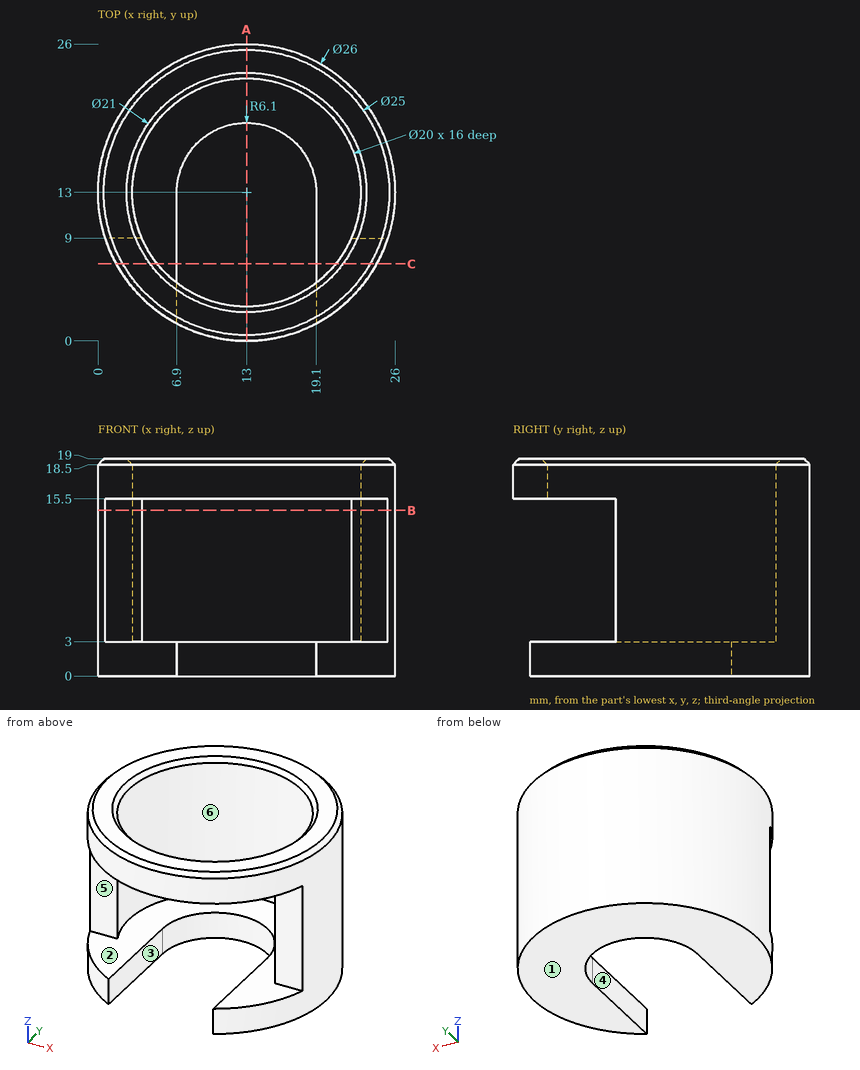
Geometry check sheet. Reference: drawing and pictorial views, mm from the part's lowest x, y, z. A direction names the side the tool comes from. Coordinates: 2 decimals unless noted, no trailing zeros. Order: outer loops, then holes, each group sorted by start corner. A loop starts at its lowest first (then second) coordinate and runs counter-clockwise, first axis right, second up. Notation, with made-up numbers: (69, 37.5) -> (127, 37.5) arc R24 ccw to (127, 54.5) -> close; hole circle Ø4 at (14.5, -30). An arc over 180 degrees is marked (long way). Put each result on its own line as item: value. Start each with the question number.
1) Material ranges on L1, parallel to X at y = 13, z = 8.5; L2, parallel to Z at x = 21.25, y = 14.5; L3, parallel to X at y = 12.5, z = 2.5, recorded low to high.
2) Cross-section at C-C (y = 6.75). State how many separate pieces and enclosed holes the cut face has, plus the area to 3 significant figures.
3) Go/stop test with flat-tipped pins: pin 1 (10 mm diameter, centred on x = 15.5, y = 13.5, fed in from +Z); pin 2 (0.9 mm diameter, centred on y = 8, z = 2, fed in from +X); pin 3 (2.5 mm diameter, centred on y = 5, z = 1.5, fed in from -X). Record where each tip stops, or that it passes through.
4) Cross-section at B-B (z = 14.5). Enter the section's corners in (x, y), plus the area to 3 significant figures.
5) Tool access check on the marked faces 4, 5 and 6. Record the directions out of +Z, -Z, +X, -X, +Y, -Y that give a thin tool (end or side, any length) a straight path to the whole face; none if there is none.
6) Release check for a two-part mould opening along Z. For the marked faces 1, 2 and 3 record: pulls with the +Z half, pulls with the -Z half, needs draft (parallel to the pull), parting line crosses it, or undercut.
7) Cross-section at A-A (x = 13). Enter the section's corners in (y, z), plus the area to 3 significant figures.
Geometry check:
1. L1: x = 0 to 3, 23 to 26
1. L2: z = 0 to 3
1. L3: x = 0.01 to 6.9, 19.1 to 25.99
2. separate pieces: 4
2. enclosed holes: 0
2. area: 56.3 mm^2
3. pin 1: stops at z = 3
3. pin 2: stops at x = 25.18
3. pin 3: stops at x = 1.89
4. outline: (0.63, 9) -> (3.83, 9) arc R10 cw (long way) to (22.17, 9) -> (25.37, 9) arc R13 ccw (long way) to start
4. area: 133 mm^2
5. face 4: -Z, -Y
5. face 5: +X, -X, -Y
5. face 6: +Z
6. face 1: pulls with the -Z half
6. face 2: undercut
6. face 3: needs draft
7. outline: (0, 15.5) -> (3, 15.5) -> (3, 18.5) -> (2.5, 19) -> (0.5, 19) -> (0, 18.5) -> close; (19.1, 0) -> (26, 0) -> (26, 18.5) -> (25.5, 19) -> (23.5, 19) -> (23, 18.5) -> (23, 3) -> (19.1, 3) -> close
7. area: 78.7 mm^2
